The model under review builds one solid part; all positions refer to its coordinate system, in mm. Coordinates: 2 decimals unless noted, no trailing zeros. Order: outer loops, then holes, each group sorted by start corner. A loop starts at its lowest first (then second) coordinate and runs counter-clockwise, first axis right, second up. Notation, with made-up numbers: M -30.5,27 L -24.5,27 A20 ccw -24.5,45 Z; hole C -16,-26.5 d2. An arc over 180 degrees is marked long. One line per item, written item: value.
```python
from build123d import *

# Parameters (mm, degrees)
SKETCH1_R           = 12.7
BOSS_EXTRUDE1_DEPTH = 8
SKETCH2_R           = 2.5
CUT_EXTRUDE1_DEPTH  = 8


with BuildPart() as part:
    # Sketch1 → Boss-Extrude1 (new body)
    with BuildSketch(Plane.XY):
        Circle(SKETCH1_R)
    extrude(amount=BOSS_EXTRUDE1_DEPTH)

    # Sketch2 → Cut-Extrude1 (cut)
    with BuildSketch(Plane.XY.offset(8)):
        with Locations((0, 10)):
            Circle(SKETCH2_R)
        with Locations((8.660254038, 5)):
            Circle(SKETCH2_R)
        with Locations((8.660254038, -5)):
            Circle(SKETCH2_R)
        with Locations((0, -10)):
            Circle(SKETCH2_R)
        with Locations((-8.660254038, -5)):
            Circle(SKETCH2_R)
        with Locations((-8.660254038, 5)):
            Circle(SKETCH2_R)
        Circle(SKETCH2_R)
    extrude(amount=-CUT_EXTRUDE1_DEPTH, mode=Mode.SUBTRACT)


solid = part.part
```
(1) For L1, parallel to Y at x = 0, z = 2.5; L2, parallel to Y at x = 10.5, z = 7.5; L3, parallel to X at y = 7, z = 2, list the stretches that pass through material, from the lowest coordinate up.
Geometry results:
L1: y = -12.7 to -12.5, -7.5 to -2.5, 2.5 to 7.5, 12.5 to 12.7
L2: y = -7.14 to -6.69, -3.31 to 3.31, 6.69 to 7.14
L3: x = -10.6 to -10.16, -7.16 to 7.16, 10.16 to 10.6
(2) We need section C-C, the plane x = 0. State the section outline as (y, z) points.
Geometry results:
outline: M -12.7,0 L -12.5,0 L -12.5,8 L -12.7,8 Z; M -7.5,0 L -2.5,0 L -2.5,8 L -7.5,8 Z; M 2.5,0 L 7.5,0 L 7.5,8 L 2.5,8 Z; M 12.5,0 L 12.7,0 L 12.7,8 L 12.5,8 Z
(3) Mouldability with a two-part tool opening along X and no side actions: class faces 1 (the cylindrical face through (-2.75, -12.4, 3.94)), 2 (the flat face through (0, -3, 0)), 3 (the cylindrical face through (-6.276, 5.751, 4.056)) as +X half, -X half, draft (parallel to the pull), parting line (faces both ways), or undercut.
Geometry results:
face 1: parting line
face 2: draft
face 3: undercut
(4) We need section D-D, the plane y = 5. State the section outline as (x, z) points.
Geometry results:
outline: M -11.67,0 L -11.16,0 L -11.16,8 L -11.67,8 Z; M -6.16,0 L 6.16,0 L 6.16,8 L -6.16,8 Z; M 11.16,0 L 11.67,0 L 11.67,8 L 11.16,8 Z
(5) Insertion check: pin 1 Ø4 at (x, y) = (8.66, 5) entering from +Z; pin 2 Ø1.5 at (x, z) = (3, 4) entering from +Y; pin 3 Ø4 at (x, z) = (4.5, 1.5) entering from -Y; pin 4 Ø2 at (y, z) = (7, 1) entering from -X. Each pin has a flat end and moves straight along its axis. Give the tip position at first contact, or say it passes through.
Geometry results:
pin 1: passes through
pin 2: stops at y = 12.5
pin 3: stops at y = -12.45
pin 4: stops at x = -11.19
(6) We need section A-A, the plane y = 0. State the section outline as (x, z) points, plus the area to 3 significant figures.
Geometry results:
outline: M -12.7,0 L -2.5,0 L -2.5,8 L -12.7,8 Z; M 2.5,0 L 12.7,0 L 12.7,8 L 2.5,8 Z
area: 163 mm2
(7) We need section B-B, the plane z = 2. State the section outline as (x, y) points, plus the area to 3 significant figures.
Geometry results:
outline: C 0,0 d25.4; hole C -8.66,-5 d5; hole C -8.66,5 d5; hole C 0,-10 d5; hole C 0,0 d5; hole C 0,10 d5; hole C 8.66,-5 d5; hole C 8.66,5 d5
area: 369 mm2
